Geometry: final body of the model. Coordinates: model frame, mm. Round coordinates to 2 decimals unless told otherwise and drop trailing zeros. Loops run counter-clockwise (first coordinate to the right, second up) from the corner with the lowest first, then second, coordinate; pieces in that order, holes last. Notation, with made-up numbers: (-6.5, 77.5) - (48.5, 77.5) arc R29 ccw to (48.5, 110.5) - close; hole circle Ø6 at (66, 62). An arc over 180 degrees is marked (long way). Answer as CSV lines item,"result".
from build123d import *

# Parameters (mm, degrees)
SKETCH_1_W               = 20
SKETCH_1_H               = 20
SKETCH_1_R               = 2
SKETCH_1_R_2             = 2.15
EXTRUDE_1_DEPTH          = 205
CUT_EXTRUDE_1_REACH      = 207.487
PATTERN_CIRCULAR_1_COUNT = 4
FILLET_1_R               = 0.3


with BuildPart() as part:
    # Sketch 1 → Extrude 1 (new body)
    with BuildSketch(Plane.XY):
        Rectangle(SKETCH_1_W, SKETCH_1_H)
        with Locations(Location((-7, 7, 0), (0, 0, 180))):
            Circle(SKETCH_1_R, mode=Mode.SUBTRACT)
        with Locations(Location((-7, -7, 0), (0, 0, 180))):
            Circle(SKETCH_1_R, mode=Mode.SUBTRACT)
        with Locations(Location((0, 0, 0), (0, 0, 180))):
            Circle(SKETCH_1_R_2, mode=Mode.SUBTRACT)
        with Locations(Location((7, 7, 0), (0, 0, 180))):
            Circle(SKETCH_1_R, mode=Mode.SUBTRACT)
        with Locations(Location((7, -7, 0), (0, 0, 180))):
            Circle(SKETCH_1_R, mode=Mode.SUBTRACT)
    extrude(amount=EXTRUDE_1_DEPTH)

    # Sketch 1_3 → Cut-Extrude 1 (cut, up to next)
    with BuildSketch(Plane.XY, mode=Mode.PRIVATE) as cut_extrude_1_sk1:
        with BuildLine():
            Line((-8.5, 2.65), (-10, 2.65))
            Line((-10, 2.65), (-10, -2.65))
            Line((-10, -2.65), (-8.5, -2.65))
            Line((-8.5, -2.65), (-8.5, -4.15))
            Line((-8.5, -4.15), (-4.503166667, -4.15))
            ThreePointArc((-4.503166667, -4.15), (-3.3, 0), (-4.503166667, 4.15))
            Line((-4.503166667, 4.15), (-8.5, 4.15))
            Line((-8.5, 4.15), (-8.5, 2.65))
        make_face()
    cut_extrude_1_tool1 = extrude(cut_extrude_1_sk1.sketch, amount=CUT_EXTRUDE_1_REACH, mode=Mode.PRIVATE) & part.part
    cut_extrude_1 = cut_extrude_1_tool1.solids().sort_by_distance((-6.606913, 0, 0))[0]
    add(cut_extrude_1, mode=Mode.SUBTRACT)

    # Pattern Circular 1: Cut-Extrude 1 ×4 about axis
    pattern_circular_1_axis = Axis((0, 0, 0), (0, 0, 1))
    for i in range(1, PATTERN_CIRCULAR_1_COUNT):
        add(cut_extrude_1.rotate(pattern_circular_1_axis, i * 360 / PATTERN_CIRCULAR_1_COUNT), mode=Mode.SUBTRACT)

    # Fillet 1
    fillet_1_edges = [part.edges().sort_by_distance(p)[0] for p in [
        (-10, -10, 102.5),
        (10, -10, 102.5),
        (10, 10, 102.5),
        (-10, 10, 102.5),
    ]]
    fillet(fillet_1_edges, radius=FILLET_1_R)


solid = part.part
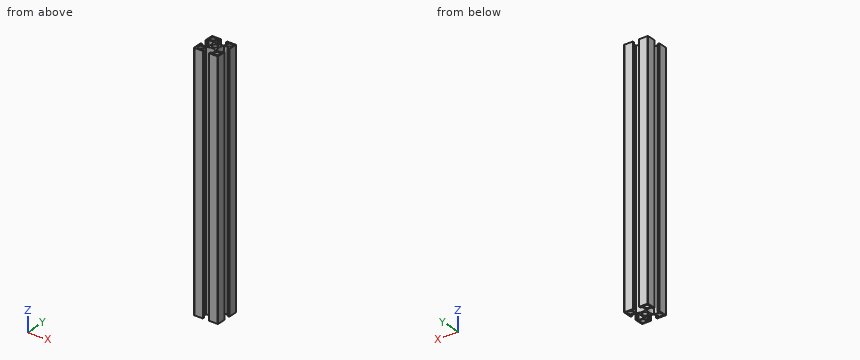
(1) Section C-C (z = 71.5). Give the number of separate pieces and of enclosed holes in the cut face, and give its area (3 significant figures).
Findings below:
separate pieces,"1"
enclosed holes,"5"
area,"144 mm2"
(2) Material intervals for line 1 along Y through (x, z) = (-7, 60.5), sorted ascending.
Findings below:
line 1,"-10 to -9, -5 to -4.15, 4.15 to 5, 9 to 10"
(3) Section A-A (x = 0). Output: boundary loops of the cut face in (y, z), and give its area (4 significant figures).
Findings below:
outline,"(-3.3, 0) - (-2.15, 0) - (-2.15, 205) - (-3.3, 205) - close; (2.15, 0) - (3.3, 0) - (3.3, 205) - (2.15, 205) - close"
area,"471.5 mm2"
